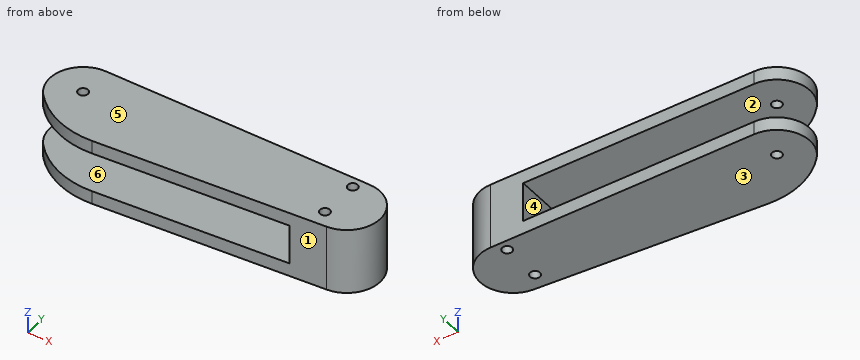
from build123d import *

# Parameters (mm, degrees)
SKETCH1_R               = 1.5
BOSS_EXTRUDE1_DEPTH     = 10
SKETCH2_W               = 140
SKETCH2_H               = 12
CUT_EXTRUDE1_DEPTH      = 11
CUT_EXTRUDE1_DEPTH_BACK = 16


with BuildPart() as part:
    # Sketch1 → Boss-Extrude1 (new body, symmetric)
    with BuildSketch(Plane.XY):
        with BuildLine():
            Line((43.628033294, 10), (0, 10))
            ThreePointArc((0, 10), (-9.128709292, 4.082482905), (-7.453559925, -6.666666667))
            ThreePointArc((-7.453559925, -6.666666667), (1.814979124, -13.179517203), (13.006384648, -14.933222025))
            Line((13.006384648, -14.933222025), (80.730417904, -9.97328881))
            ThreePointArc((80.730417904, -9.97328881), (89.993319971, 0.365453076), (80, 10))
            Line((80, 10), (43.628033294, 10))
        make_face()
        with Locations((77, -5.283013816)):
            Circle(SKETCH1_R, mode=Mode.SUBTRACT)
        with Locations((77, 6.904943152)):
            Circle(SKETCH1_R, mode=Mode.SUBTRACT)
        Circle(SKETCH1_R, mode=Mode.SUBTRACT)
    extrude(amount=BOSS_EXTRUDE1_DEPTH, both=True)

    # Sketch2 → Cut-Extrude1 (cut, two sides)
    with BuildSketch(Plane(origin=(0, 0, 0), x_dir=(1, 0, 0), z_dir=(0, 1, 0))) as cut_extrude1_sk:
        Rectangle(SKETCH2_W, SKETCH2_H)
    extrude(amount=CUT_EXTRUDE1_DEPTH, mode=Mode.SUBTRACT)
    extrude(cut_extrude1_sk.sketch, amount=-CUT_EXTRUDE1_DEPTH_BACK, mode=Mode.SUBTRACT)


solid = part.part
For this review, take the finished solid that the model builds, in its own axes (mm). Face numbers are marked on the shaded views. A direction names the side the tool comes from. Round coordinates to 2 decimals unless told otherwise and drop trailing zeros. Write each loop counter-clockwise with the first axis right and the second up, starting at its lowest first coordinate (ties: lowest second). Pieces come first, ordered by that corner, then holes. Notation, with made-up numbers: (63.5, 37) - (93.5, 37) arc R21 ccw to (93.5, 45) - close; hole circle Ø5 at (85, 49). An arc over 180 degrees is marked (long way). Use a Markdown table: item, result.
Q1. The part is to be moulded in two halves that separate along Z. For the marked faces 3, 4, 5 and 6, say which applies: pulls with the +Z half, pulls with the -Z half, needs draft (parallel to the pull), parting line crosses it, or undercut.
Derived:
| item | result |
|---|---|
| face 3 | pulls with the -Z half |
| face 4 | undercut |
| face 5 | pulls with the +Z half |
| face 6 | undercut |
Q2. Machinability: for the marked faces 1 and 2, which of the approach directions +Z, -Z, +X, -X, +Y, -Y give a long, thin tool a straight path to every point of the face, cutting with its end or side? Answer none if there is none.
Derived:
| item | result |
|---|---|
| face 1 | +Z, -Z, +X, -Y |
| face 2 | -X, +Y, -Y |
Q3. We need section A-A (x = 67.5). Give the boundary of the cut face in (y, z), plus the area to 3 significant figures.
Derived:
| item | result |
|---|---|
| outline | (-10.94, -10) - (10, -10) - (10, -6) - (-10.94, -6) - close; (-10.94, 6) - (10, 6) - (10, 10) - (-10.94, 10) - close |
| area | 168 mm2 |
Q4. Clearance check with flat-ended pins moving along their axes: pin 1 (5 mm diameter, centred on x = 77, y = 6.9, fed in from +Z); pin 2 (1.5 mm diameter, centred on y = -6, z = 4.5, fed in from -X); pin 3 (8 mm diameter, centred on x = 15, z = -7, fed in from -Y). State where each tip first meets the part, or that it passes through.
Derived:
| item | result |
|---|---|
| pin 1 | stops at z = 10 |
| pin 2 | stops at x = 70 |
| pin 3 | stops at y = -15 |
Q5. Wall thickness on line 1 along Z through (x, y) = (0.5, 3.25); line 2 along Y through (x, z) = (77, 2); line 3 along X through (y, z) = (-4, 5.5): over which ranges is each line inside the solid? List them lowest first.
Derived:
| item | result |
|---|---|
| line 1 | z = -10 to -6, 6 to 10 |
| line 2 | y = -10.25 to -6.78, -3.78 to 5.4, 8.4 to 10 |
| line 3 | x = 70 to 76.22, 77.78 to 89.17 |
Q6. We need section B-B (y = -12.5). Give the boundary of the cut face in (x, z).
Derived:
| item | result |
|---|---|
| outline | (0.28, -10) - (46.23, -10) - (46.23, -6) - (0.28, -6) - close; (0.28, 6) - (46.23, 6) - (46.23, 10) - (0.28, 10) - close |
Q7. We need section D-D (z = -4). Give the boundary of the cut face in (x, y).
Derived:
| item | result |
|---|---|
| outline | (70, -10.76) - (80.73, -9.97) arc R10 ccw to (80, 10) - (70, 10) - close; hole circle Ø3 at (77, -5.28); hole circle Ø3 at (77, 6.9) |
Q8. We need section C-C (z = 8.5). Give the boundary of the cut face in (x, y).
Derived:
| item | result |
|---|---|
| outline | (-7.45, -6.67) arc R25 ccw to (13.01, -14.93) - (80.73, -9.97) arc R10 ccw to (80, 10) - (0, 10) arc R10 ccw to start; hole circle Ø3 at (0, 0); hole circle Ø3 at (77, -5.28); hole circle Ø3 at (77, 6.9) |
